Check sheet for the modelled part. Datum: model origin and axes. Units: mm. Face numbers are marked on the shaded views. A direction names the side the tool comes from. Give positions to 0.01 mm unless a question says otherwise; leave off trailing zeros. Loops run counter-clockwise (first coordinate to the right, second up) from the corner with the lowest first, then second, coordinate; pieces in that order, holes last. Notation, with made-up numbers: (63, -30.5) - (99, -30.5) arc R10 ccw to (99, -21.5) - close; hole circle Ø11 at (36.5, 56). An arc over 180 degrees is marked (long way). Use one line per item in the form item = value.
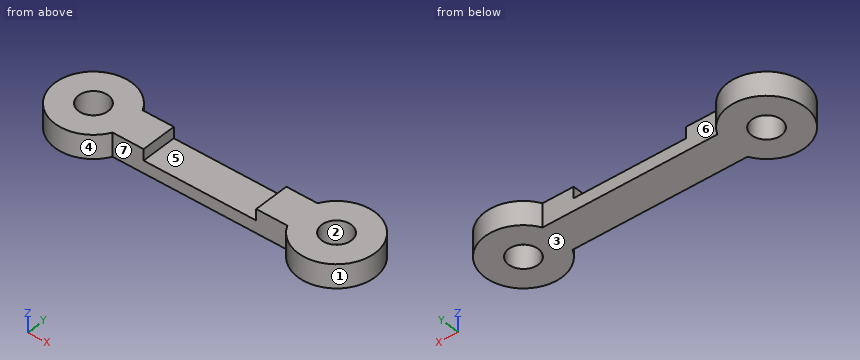
from build123d import *

# Parameters (mm, degrees)
SKETCH_R     = 2.5
PAD_DEPTH    = 4
SKETCH001_W  = 19
SKETCH001_H  = 6
POCKET_DEPTH = 1.9


with BuildPart() as part:
    # Sketch → Pad (new body)
    with BuildSketch(Plane.XY):
        with BuildLine():
            Line((-14.75, 3), (14.75, 3))
            ThreePointArc((14.75, -3), (27.016281, 0), (14.75, 3))
            Line((14.75, -3), (-14.75, -3))
            ThreePointArc((-14.75, 3), (-27.016281, 0), (-14.75, -3))
        make_face()
        with Locations((-20.516281, 0)):
            Circle(SKETCH_R, mode=Mode.SUBTRACT)
        with Locations((20.516281, 0)):
            Circle(SKETCH_R, mode=Mode.SUBTRACT)
    extrude(amount=PAD_DEPTH)

    # Sketch001 → Pocket (cut)
    with BuildSketch(Plane.XY.offset(4)):
        Rectangle(SKETCH001_W, SKETCH001_H)
    extrude(amount=-POCKET_DEPTH, mode=Mode.SUBTRACT)


solid = part.part
Item 1: Access from +Z, -Z, +X, -X, +Y, -Y to the whole of each face (thin tool, end or side, straight path). Record for the marked faces 4, 5, 6 and 7.
Answer block:
face_4 = +Z, -Z
face_5 = +Z, +Y, -Y
face_6 = +Z, -Z, +Y
face_7 = +Z, -Z, -Y
Item 2: Gauge pin test, flat ends, axial feed: P1, Ø1, axis at y = -1.5, z = 3.5, coming from the +X side; P2, Ø1.8, axis at x = 1.5, y = 1, coming from the +Z side; P3, Ø1.5, axis at y = -5, z = 2.5, coming from the -X side. Record the tip position at first contact, or that the pin passes through.
Answer block:
P1 = 26.94
P2 = 2.1
P3 = -25.43
Item 3: Thickness scan on L1, parallel to X at y = 1, z = 2.85 (3 decimals); L2, parallel to X at y = -2, z = 2.5; L3, parallel to X at y = -1.5, z = 2. Record the ranges inside material, lowest first.
Answer block:
L1 = -26.939 to -22.808, -18.225 to -9.5, 9.5 to 18.225, 22.808 to 26.939
L2 = -26.7 to -22.02, -19.02 to -9.5, 9.5 to 19.02, 22.02 to 26.7
L3 = -26.84 to -22.52, -18.52 to 18.52, 22.52 to 26.84
Item 4: Section check A-A on y = 0. Record the boundary of the cut face in (x, z), then the cut area to 3 significant figures.
Answer block:
outline = (-27.02, 0) - (-23.02, 0) - (-23.02, 4) - (-27.02, 4) - close; (-18.02, 0) - (18.02, 0) - (18.02, 4) - (9.5, 4) - (9.5, 2.1) - (-9.5, 2.1) - (-9.5, 4) - (-18.02, 4) - close; (23.02, 0) - (27.02, 0) - (27.02, 4) - (23.02, 4) - close
area = 140 mm2
Item 5: Mould release check, pull along Y, two halves, no side actions. Record for the marked faces 1, 2 and 3: released by +Y, released by -Y, zero draft, split by the parting line, or undercut.
Answer block:
face_1 = split by the parting line
face_2 = undercut
face_3 = zero draft
Item 6: Section check C-C on x = 22. Record the boundary of the cut face in (y, z), then the cut area to 3 significant figures.
Answer block:
outline = (-6.33, 0) - (-2.01, 0) - (-2.01, 4) - (-6.33, 4) - close; (2.01, 0) - (6.33, 0) - (6.33, 4) - (2.01, 4) - close
area = 34.5 mm2
Item 7: Section check D-D on y = -4.75. Record the boundary of the cut face in (x, z), then the cut area to 3 significant figures.
Answer block:
outline = (-24.95, 0) - (-16.08, 0) - (-16.08, 4) - (-24.95, 4) - close; (16.08, 0) - (24.95, 0) - (24.95, 4) - (16.08, 4) - close
area = 71.0 mm2
Item 8: Section check B-B on z = 2.85. Record the boundary of the cut face in (x, y), then the cut area to 3 significant figures.
Answer block:
outline = (-14.75, -3) - (-9.5, -3) - (-9.5, 3) - (-14.75, 3) arc R6.5 ccw (long way) to start; (9.5, -3) - (14.75, -3) arc R6.5 ccw (long way) to (14.75, 3) - (9.5, 3) - close; hole circle Ø5 at (-20.52, 0); hole circle Ø5 at (20.52, 0)
area = 283 mm2
